Verification items for this drawing (mm, ordinates from the low corner). A direction names the side the tool comes from. Give positions to 0.01 mm unless a question says otherwise; leave off trailing zeros. Loops run counter-clockwise (first coordinate to the right, second up) from the corner with the lowest first, then second, coordinate; pieces in that order, holes last. Notation, with made-up numbers: (-9.5, 73) -> (22.5, 73) arc R30 ccw to (22.5, 100) -> close; hole circle Ø8 at (60.5, 25.25). An arc over 180 degrees is marked (long way). Answer in a Markdown table with one row per item. Add a question column.
Q1. Set-up check for the marked faces 4 and 5: record each of +Z, -Z, +X, -X, +Y, -Y from which the full face is reachable in a straight line by a thin tool's end or side.
Q2. Section check D-D on x = 13.5. Enter the section's corners in (y, z).
Q3. Section check A-A on x = 43.5. Enter the section's corners in (y, z), and give its area (3 significant figures).
Q4. Section check C-C on z = 17. Give the number of separate pieces and of enclosed holes in the cut face, and give its area (3 significant figures).
Q5. Release check for a two-part mould opening along Y. For the marked faces 1, 2 and 3 record: pulls with the +Y half, pulls with the -Y half, needs draft (parallel to the pull), parting line crosses it, or undercut.
Q6. Gauge pin test, flat ends, axial feed: P1, Ø16, axis at x = 19, z = 23, coming from the -Y side; P2, Ø1.5, axis at x = 12.5, y = 16, coming from the +Z side; P3, Ø3, axis at x = 13, y = 8.5, coming from the +Z side. Record the tip position at first contact, or that the pin passes through.
Q7. Section check B-B on y = 21. Enter the section's corners in (x, z) (3 decimals), and give its area (3 significant figures).
Q8. Material ranges on probe 1 along X at (y, z) = (1.55, 17); probe 2 along Y at (x, z) = (22, 25); probe 3 along Y at (x, z) = (18, 1.8) (3 decimals), recorded low to high.
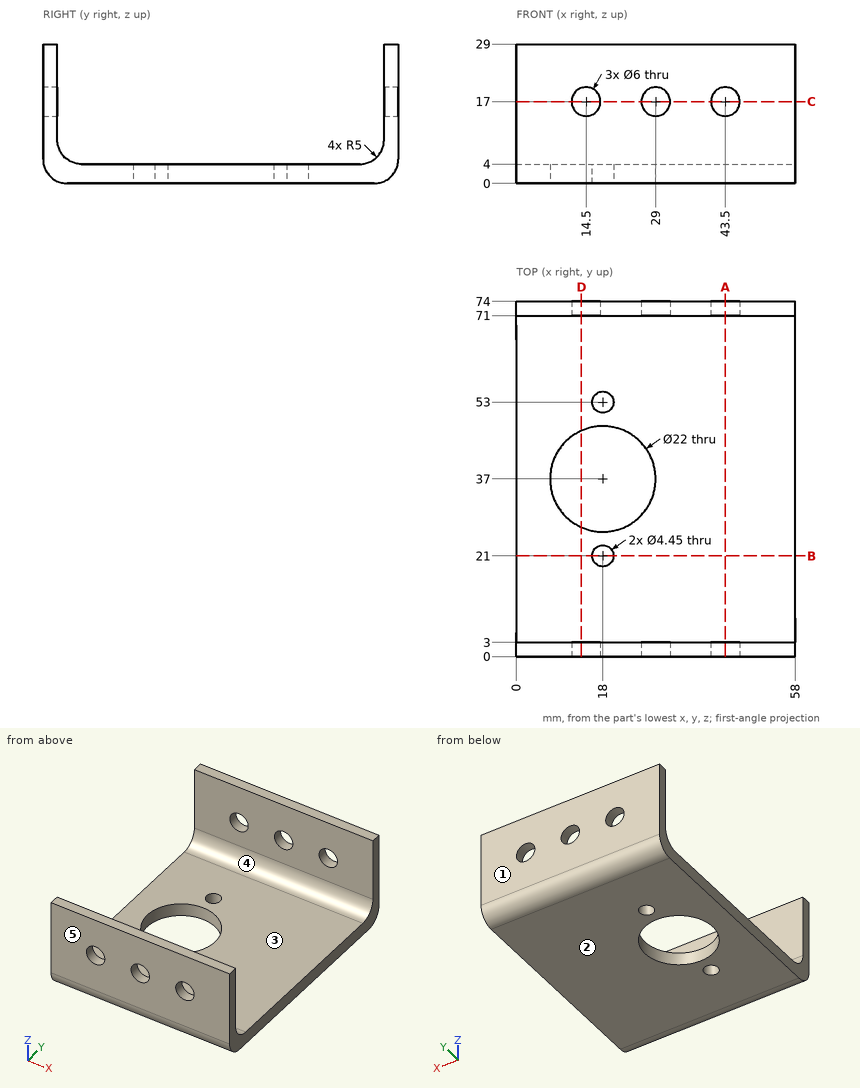
Taken from the geometry:
| question | item | result |
|---|---|---|
| 1 | face 4 | +Z, +X, -X |
| 1 | face 5 | +Z, -Z, +X, -X, -Y |
| 2 | outline | (0, 5) arc R5 ccw to (5, 0) -> (26.96, 0) -> (26.96, 4) -> (8, 4) arc R5 cw to (3, 9) -> (3, 14.17) -> (0, 14.17) -> close; (0, 19.83) -> (3, 19.83) -> (3, 29) -> (0, 29) -> close; (47.04, 0) -> (69, 0) arc R5 ccw to (74, 5) -> (74, 14.17) -> (71, 14.17) -> (71, 9) arc R5 cw to (66, 4) -> (47.04, 4) -> close; (71, 19.83) -> (74, 19.83) -> (74, 29) -> (71, 29) -> close |
| 3 | outline | (0, 5) arc R5 ccw to (5, 0) -> (69, 0) arc R5 ccw to (74, 5) -> (74, 14) -> (71, 14) -> (71, 9) arc R5 cw to (66, 4) -> (8, 4) arc R5 cw to (3, 9) -> (3, 14) -> (0, 14) -> close; (0, 20) -> (3, 20) -> (3, 29) -> (0, 29) -> close; (71, 20) -> (74, 20) -> (74, 29) -> (71, 29) -> close |
| 3 | area | 410 mm² |
| 4 | separate pieces | 8 |
| 4 | enclosed holes | 0 |
| 4 | area | 240 mm² |
| 5 | face 1 | pulls with the +Y half |
| 5 | face 2 | needs draft |
| 5 | face 3 | undercut |
| 6 | P1 | stops at y = 0 |
| 6 | P2 | stops at z = 4 |
| 6 | P3 | stops at z = 4.1 |
| 7 | outline | (0, 0) -> (15.775, 0) -> (15.775, 4) -> (0, 4) -> close; (20.225, 0) -> (58, 0) -> (58, 4) -> (20.225, 4) -> close |
| 7 | area | 214 mm² |
| 8 | probe 1 | x = 0 to 11.5, 17.5 to 26, 32 to 40.5, 46.5 to 58 |
| 8 | probe 2 | y = 0 to 3, 71 to 74 |
| 8 | probe 3 | y = 1.158 to 18.775, 23.225 to 26, 48 to 50.775, 55.225 to 72.842 |
